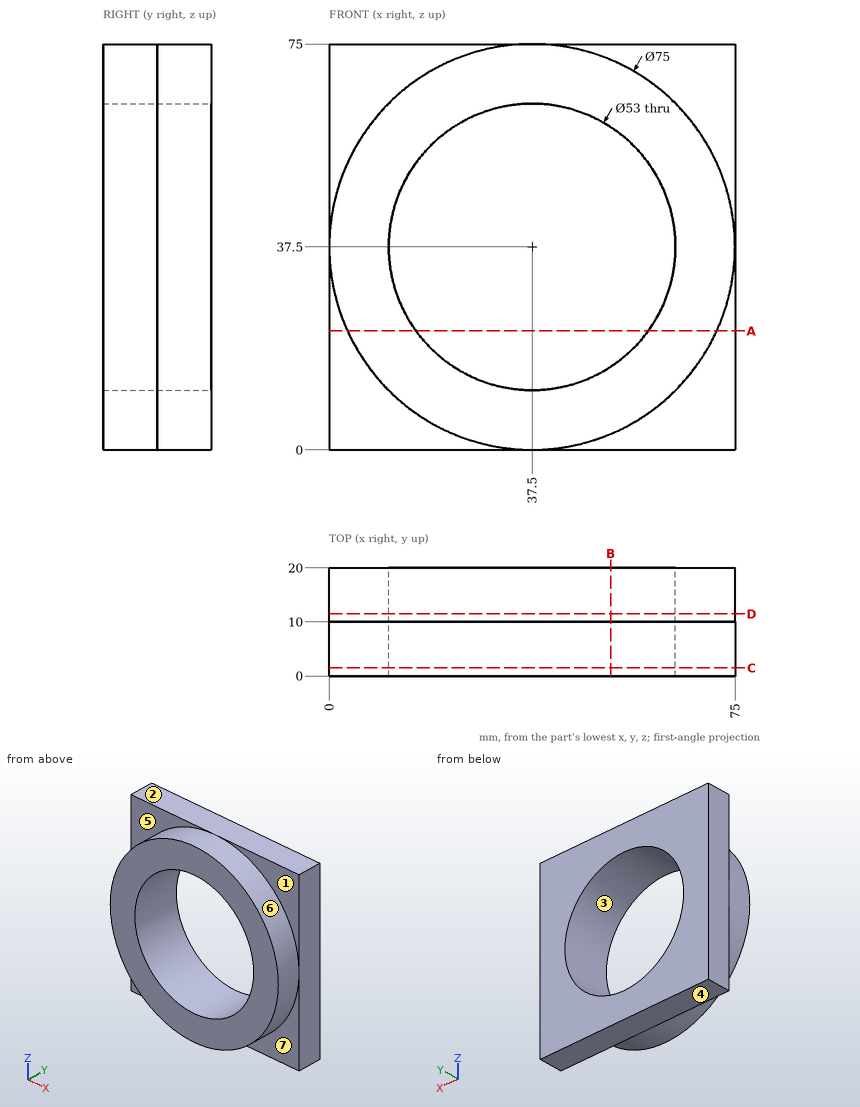
Input: dimensioned drawing with shaded views. Units: mm. Origin: part minimum x, y, z. A direction names the side the tool comes from. Give positions to 0.01 mm unless a question says otherwise; leave off trailing zeros. Write each loop counter-clockwise with the first axis right and the second up, starting at its lowest first coordinate (ties: lowest second). Pieces come first, ordered by that corner, then holes.
Q1. First-contact query: P1, Ø8, axis at x = 60.5, y = 10.5, coming from the -Z side; P2, Ø1.5, axis at y = 5, z = 41.5, coming from the -X side. Flat tips, straight axial feed; report the tip coordinate or a pass-through.
Q2. Section A-A, the plane z = 22. Output: boundary loops of the cut face in (x, y).
Q3. Pull-direction query (Z, two-part tool) for the marked faces 1, 2, 3 and 4; classes: pulls with the +Z half, pulls with the -Z half, needs draft (parallel to the pull), parting line crosses it, or undercut.
Q4. Section D-D, the plane y = 11.5. Output: boundary loops of the cut face in (x, z), plus the area to 3 significant figures.
Q5. Set-up query: the marked faces 5, 6 and 7. Return all of +Z, -Z, +X, -X, +Y, -Y with unobstructed straight access to the full face (end or side cutting, diameter ignored); none if empty.
Q6. Section B-B, the plane x = 52. Output: boundary loops of the cut face in (y, z), plus the area to 3 significant figures.
Q7. Section C-C, the plane y = 1.5. Output: boundary loops of the cut face in (x, z), plus the area to 3 significant figures.
Q8. Material intervals for probe 1 along Z at (x, y) = (37, 4.5); probe 2 along Z at (x, y) = (45.5, 18.5), sorted ascending.
Filled in:
1. P1: stops at z = 0
1. P2: stops at x = 0.14
2. outline: (0, 10) - (3.35, 10) - (3.35, 0) - (16.01, 0) - (16.01, 20) - (0, 20) - close; (58.99, 0) - (71.65, 0) - (71.65, 10) - (75, 10) - (75, 20) - (58.99, 20) - close
3. face 1: needs draft
3. face 2: pulls with the +Z half
3. face 3: undercut
3. face 4: pulls with the -Z half
4. outline: (0, 0) - (75, 0) - (75, 75) - (0, 75) - close; hole circle Ø53 at (37.5, 37.5)
4. area: 3,420 mm2
5. face 5: +Z, -X, -Y
5. face 6: -Y
5. face 7: -Z, +X, -Y
6. outline: (0, 2.92) - (10, 2.92) - (10, 0) - (20, 0) - (20, 15.32) - (0, 15.32) - close; (0, 59.68) - (20, 59.68) - (20, 75) - (10, 75) - (10, 72.08) - (0, 72.08) - close
6. area: 554 mm2
7. outline: circle Ø75 at (37.5, 37.5); hole circle Ø53 at (37.5, 37.5)
7. area: 2,210 mm2
8. probe 1: z = 0 to 11, 64 to 75
8. probe 2: z = 0 to 12.24, 62.76 to 75
